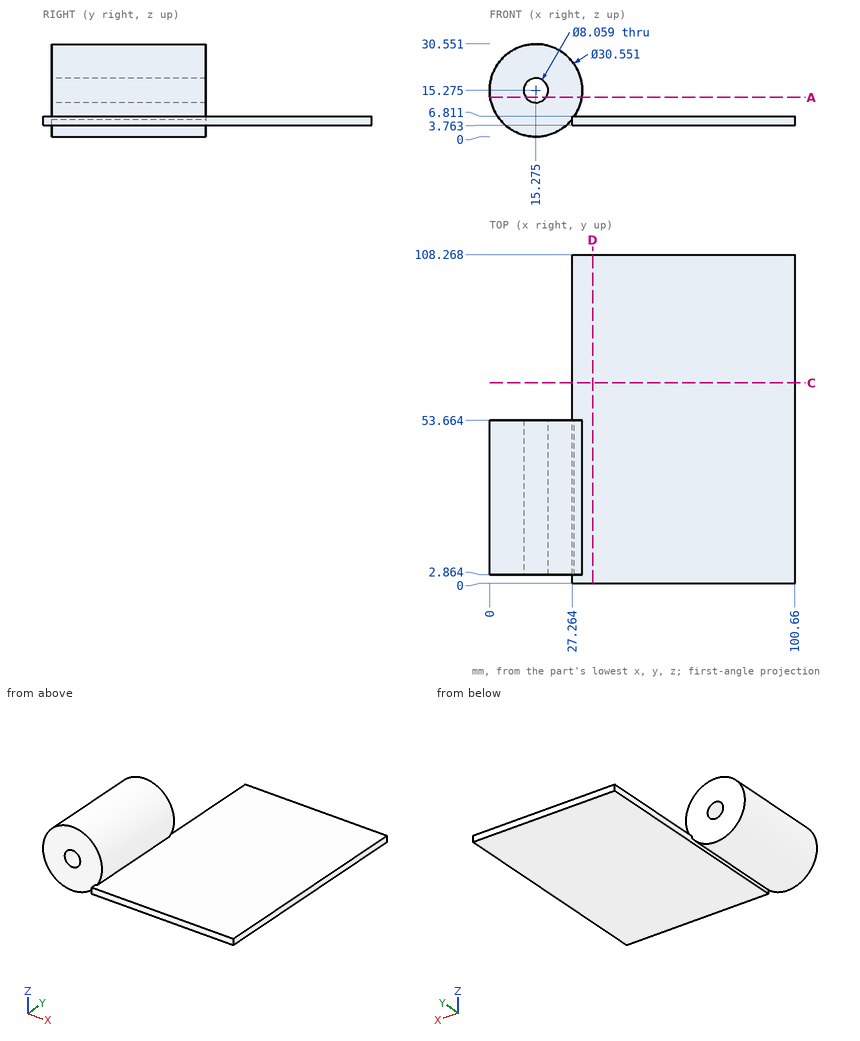
Answer from the drawing. Dimensions are ordinates in mm from the lowest x, y and z of the part. Round coordinates to 2 decimals unless told otherwise and drop trailing zeros. Loops run counter-clockwise (first coordinate to the right, second up) from the corner with the lowest first, then second, coordinate; pieces in that order, holes last.
Q1. Each of these flat-tipped pins is pushed along its axis until it touches: pin 1 (2 mm diameter, centred on y = 44.5, z = 11.5, fed in from +X); pin 2 (3 mm diameter, centred on x = 23.5, y = 35, fed in from +Z); pin 3 (3 mm diameter, centred on x = 77, y = 32, fed in from +Z); pin 4 (8 mm diameter, centred on y = 95, z = 8, fed in from +X). Where does it stop, or does it pass through?
Q2. Section C-C on y = 66 is taken. Write down the section's boundary in (x, z) (1 decimal), and give its area (3 significant figures).
Q3. Section D-D on x = 34 is taken. Write down the section's boundary in (y, z).
Q4. Section A-A on z = 13 is taken. Write down the section's boundary in (x, y).
Q5. Consider probe 1 along X at (y, z) = (73.5, 4) (1 decimal); probe 2 along Z at (x, y) = (35, 37.5); probe 3 along Y at (x, z) = (7, 4). Determine where each line is inside the solid, lowest interval first.
Output:
1. pin 1: stops at x = 30.3
1. pin 2: stops at z = 28.99
1. pin 3: stops at z = 6.81
1. pin 4: stops at x = 100.66
2. outline: (27.3, 3.8) - (100.7, 3.8) - (100.7, 6.8) - (27.3, 6.8) - close
2. area: 224 mm2
3. outline: (0, 3.76) - (108.27, 3.76) - (108.27, 6.81) - (0, 6.81) - close
4. outline: (0.17, 2.86) - (11.95, 2.86) - (11.95, 53.66) - (0.17, 53.66) - close; (18.6, 2.86) - (30.38, 2.86) - (30.38, 53.66) - (18.6, 53.66) - close
5. probe 1: x = 27.3 to 100.7
5. probe 2: z = 3.76 to 6.81
5. probe 3: y = 2.86 to 53.66
